Geometry check sheet. Reference: the model listing, model coordinates, mm. A direction names the side the tool comes from. Coordinates: 2 decimals unless noted, no trailing zeros. Loops run counter-clockwise (first coordinate to the right, second up) from the corner with the lowest first, then second, coordinate; pieces in that order, holes last.
from build123d import *

# Parameters (mm, degrees)
F0_R     = 0.4
F1_DEPTH = 4
F2_R     = 0.4
F3_DEPTH = 2.5
F4_R     = 2
F5_DEPTH = 0.5
F6_R     = 1.75
F7_DEPTH = 5
F8_R     = 0.4
F9_DEPTH = 4


with BuildPart() as f1:
    # F0 (on Top) → F1 (new body)
    with BuildSketch(Plane.XY):
        Circle(F0_R)
    extrude(amount=F1_DEPTH)

    # F2 (on face) → F3 (join)
    with BuildSketch(Plane.XY.offset(4)):
        Polygon((1.6, -0.92376), (1.6, 0.92376), (0, 1.847521), (-1.6, 0.92376), (-1.6, -0.92376), (0, -1.847521), align=None)
        Circle(F2_R, mode=Mode.SUBTRACT)
        Circle(F2_R)
    extrude(amount=F3_DEPTH)

    # F4 (on face) → F5 (join)
    with BuildSketch(Plane.XY.offset(6.5)):
        Circle(F4_R)
    extrude(amount=F5_DEPTH)

    # F6 (on face) → F7 (join)
    with BuildSketch(Plane.XY.offset(7)):
        Circle(F6_R)
    extrude(amount=F7_DEPTH)

    # F8 (on face) → F9 (join)
    with BuildSketch(Plane.XY.offset(12)):
        Circle(F8_R)
    extrude(amount=F9_DEPTH)


solid = f1.part
1) Section check A-A on y = 0. Record the cut outline in (x, z), and give its area (3 significant figures).
Data:
outline: (-2, 6.5) - (-1.6, 6.5) - (-1.6, 4) - (-0.4, 4) - (-0.4, 0) - (0.4, 0) - (0.4, 4) - (1.6, 4) - (1.6, 6.5) - (2, 6.5) - (2, 7) - (1.75, 7) - (1.75, 12) - (0.4, 12) - (0.4, 16) - (-0.4, 16) - (-0.4, 12) - (-1.75, 12) - (-1.75, 7) - (-2, 7) - close
area: 33.9 mm2
2) Material ranges on probe 1 along Z at (x, y) = (-1.45, 0.2); probe 2 along Z at (x, y) = (0.15, -1.8); probe 3 along X at (y, z) = (0.9, 5.75), recorded low to high.
Data:
probe 1: z = 4 to 12
probe 2: z = 6.5 to 7
probe 3: x = -1.6 to 1.6
3) Access from +Z, -Z, +X, -X, +Y, -Y to the whole of each face (thin tool, end or side, straight path). Record for faces 1 (the flat face through (1.6, 0, 5)), 2 (the flat face through (-0.4, -0.4, 4)), 3 (the flat face through (-1.6, 0, 5)), 4 (the flat face through (-0.79, 1.39, 5.23)), 5 (the flat face through (-0.81, -1.38, 5.23)).
Data:
face 1: -Z, +X, +Y, -Y
face 2: -Z
face 3: -Z, -X, +Y, -Y
face 4: -Z, -X, +Y
face 5: -Z, -X, -Y
4) Section check B-B on z = 9. Record the cut outline in (x, y).
Data:
outline: circle Ø3.5 at (0, 0)
5) Depth check by flat-ended pin: pin 1 (1.5 mm diameter, centred on x = 1.5, z = 10.5, fed in from +Y); pin 2 (0.6 mm diameter, centred on y = 0, z = 5.5, fed in from +X); pin 3 (0.6 mm diameter, centred on y = 0, z = 5, fed in from -X); pin 4 (1.5 mm diameter, centred on y = -1.5, z = 13, fed in from +X). Enter the tip coordinate at first touch or a pass-through.
Data:
pin 1: stops at y = 1.58
pin 2: stops at x = 1.6
pin 3: stops at x = -1.6
pin 4: passes through
6) Section check C-C on x = 1.35. Record the cut outline in (y, z), and give its area (3 significant figures).
Data:
outline: (-1.48, 6.5) - (-1.07, 6.5) - (-1.07, 4) - (1.07, 4) - (1.07, 6.5) - (1.48, 6.5) - (1.48, 7) - (1.11, 7) - (1.11, 12) - (-1.11, 12) - (-1.11, 7) - (-1.48, 7) - close
area: 18.0 mm2
7) Section check D-D on y = 0.75. Record the cut outline in (x, z).
Data:
outline: (-1.85, 6.5) - (-1.6, 6.5) - (-1.6, 4) - (1.6, 4) - (1.6, 6.5) - (1.85, 6.5) - (1.85, 7) - (1.58, 7) - (1.58, 12) - (-1.58, 12) - (-1.58, 7) - (-1.85, 7) - close
